```python
from build123d import *

# Parameters (mm, degrees)
SKETCH_1_R            = 1.5
EXTRUDE_1_DEPTH       = 2
SKETCH_2_R            = 0.9
SKETCH_2_W            = 62
SKETCH_2_H            = 52
CUT_EXTRUDE_1_DEPTH   = 52.264022472
EXTRUDE_START         = -2
EXTRUDE_1_2_OUTLINE_W = 34
EXTRUDE_1_2_OUTLINE_H = 16
EXTRUDE_1_2_DEPTH     = 2
SKETCH_4_R            = 3
CUT_EXTRUDE_2_DEPTH   = 52.264022472
FILLET_1_R            = 1


# Read off the part's stored shape, not the designer's step: 拉伸-薄壁1
with BuildPart() as part:
    # 草图1 → Extrude 1 (new body)
    with BuildSketch(Plane(origin=(0, 0, 0), x_dir=(1, 0, 0), z_dir=(0, 1, 0))):
        Polygon((-37, 32), (-37, 22.5), (-40, 22.5), (-40, 7.5), (-37, 7.5), (-37, -7.5), (-40, -7.5), (-40, -22.5), (-37, -22.5), (-37, -32), (37, -32), (37, -22.5), (40, -22.5), (40, -7.5), (37, -7.5), (37, 7.5), (40, 7.5), (40, 22.5), (37, 22.5), (37, 32), align=None)
        with Locations(Location((-24.5, 29, 0), (0, 0, 270))):
            Circle(SKETCH_1_R, mode=Mode.SUBTRACT)
        with Locations(Location((24.5, 29, 0), (0, 0, 90))):
            Circle(SKETCH_1_R, mode=Mode.SUBTRACT)
        with Locations(Location((24.5, -29, 0), (0, 0, 270))):
            Circle(SKETCH_1_R, mode=Mode.SUBTRACT)
        with Locations(Location((-24.5, -29, 0), (0, 0, 90))):
            Circle(SKETCH_1_R, mode=Mode.SUBTRACT)
    extrude(amount=EXTRUDE_1_DEPTH)

    # 草图2 → 切除-拉伸1 (cut, through all)
    with BuildSketch(Plane(origin=(0, 2, 0), x_dir=(1, 0, 0), z_dir=(0, 1, 0))):
        with Locations((-37, 23.4)):
            Circle(SKETCH_2_R)
        with Locations((-37, 6.6)):
            Circle(SKETCH_2_R)
        with Locations((37, 6.6)):
            Circle(SKETCH_2_R)
        with Locations((37, 23.4)):
            Circle(SKETCH_2_R)
        with Locations((37, -23.4)):
            Circle(SKETCH_2_R)
        with Locations((-37, -23.4)):
            Circle(SKETCH_2_R)
        with Locations((37, -6.6)):
            Circle(SKETCH_2_R)
        with Locations((-37, -6.6)):
            Circle(SKETCH_2_R)
        Rectangle(SKETCH_2_W, SKETCH_2_H)
    extrude(amount=-CUT_EXTRUDE_1_DEPTH, mode=Mode.SUBTRACT)

    # Extrude 1 2 outline → Extrude 1 2 (add)
    with BuildSketch(Plane(origin=(0, 2, 0), x_dir=(1, 0, 0), z_dir=(0, 1, 0)).offset(EXTRUDE_START)):
        Polygon((-31, 26), (-31, 22.666666667), (-21, 9.333333333), (-21, -9.333333333), (-31, -22.666666667), (-31, -26), (-28.5, -26), (-18, -12), (18, -12), (28.5, -26), (31, -26), (31, -22.666666667), (21, -9.333333333), (21, 9.333333333), (31, 22.666666667), (31, 26), (28.5, 26), (18, 12), (-18, 12), (-28.5, 26), align=None)
        Rectangle(EXTRUDE_1_2_OUTLINE_W, EXTRUDE_1_2_OUTLINE_H, mode=Mode.SUBTRACT)
    extrude(amount=EXTRUDE_1_2_DEPTH)

    # 草图4 → 切除-拉伸2 (cut, through all)
    with BuildSketch(Plane(origin=(0, 2, 0), x_dir=(1, 0, 0), z_dir=(0, 1, 0))):
        with Locations((-32.5, 17.8)):
            Circle(SKETCH_4_R)
        with Locations((32.5, 17.8)):
            Circle(SKETCH_4_R)
    extrude(amount=-CUT_EXTRUDE_2_DEPTH, mode=Mode.SUBTRACT)

    # 圆角1
    fillet_1_edges = [part.edges().sort_by_distance(p)[0] for p in [
        (-31, 1, -15.201923789),
        (-31, 1, -20.398076211),
        (31, 1, -20.398076211),
        (31, 1, -15.201923789),
        (37, 1, -32),
        (40, 1, -22.5),
        (40, 1, -7.5),
        (40, 1, 7.5),
        (40, 1, 22.5),
        (37, 1, 32),
        (-37, 1, 32),
        (-40, 1, 22.5),
        (-40, 1, 7.5),
        (-40, 1, -7.5),
        (-40, 1, -22.5),
        (-37, 1, -32),
    ]]
    fillet(fillet_1_edges, radius=FILLET_1_R)


solid = part.part
```
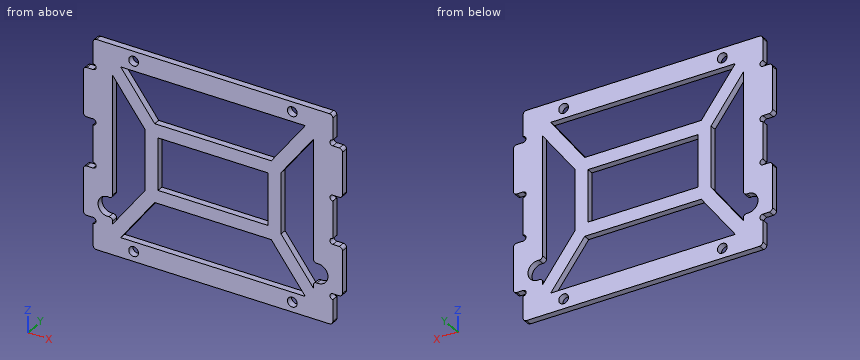
For this review, take the finished solid that the model builds, in its own axes (mm). Round coordinates to 2 decimals unless told otherwise and drop trailing zeros. Loops run counter-clockwise (first coordinate to the right, second up) from the corner with the lowest first, then second, coordinate; pieces in that order, holes last.
(1) We need section C-C (x = -27.5). Give the boundary of the cut face in (y, z).
Returned:
outline: (0, -32) - (2, -32) - (2, -26) - (0, -26) - close; (0, -24.67) - (2, -24.67) - (2, -18) - (0, -18) - close; (0, 18) - (2, 18) - (2, 24.67) - (0, 24.67) - close; (0, 26) - (2, 26) - (2, 32) - (0, 32) - close
(2) We need section B-B (z = 6.6). Give the boundary of the cut face in (x, y).
Returned:
outline: (-36.1, 0) - (-31, 0) - (-31, 2) - (-36.1, 2) - close; (-21, 0) - (-17, 0) - (-17, 2) - (-21, 2) - close; (17, 0) - (21, 0) - (21, 2) - (17, 2) - close; (31, 0) - (36.1, 0) - (36.1, 2) - (31, 2) - close
(3) Wall thickness on line 1 along Z through (x, y) = (18, 0.8); line 2 along Z through (x, y) = (6.5, 1.4); line 3 along X through (y, z) = (1, -29): over which ranges is each line inside the solid? List them lowest first.
Returned:
line 1: z = -32 to -26, -12 to 12, 26 to 32
line 2: z = -32 to -26, -12 to -8, 8 to 12, 26 to 32
line 3: x = -37 to -26, -23 to 23, 26 to 37
(4) Clearance check with flat-ended pins moving along their axes: P1, Ø1, axis at x = -38.5, y = 1.5, coming from the +Z side; P2, Ø1, axis at y = 1.5, z = 1.5, coming from the +X side; P3, Ø1, axis at x = -38, y = 0.5, coming from the -Z side. State where each tip first meets the part, or that it passes through.
Returned:
P1: stops at z = 22.5
P2: stops at x = 37
P3: stops at z = -22.5
(5) We need section D-D (y = 0.5). State how many separate pieces and enclosed holes the cut face has, plus the area to 3 significant figures.
Returned:
separate pieces: 1
enclosed holes: 9
area: 2,340 mm2
(6) We need section A-A (z = 29). Give the boundary of the cut face in (x, y), plus the area to 3 significant figures.
Returned:
outline: (-37, 0) - (-26, 0) - (-26, 2) - (-37, 2) - close; (-23, 0) - (23, 0) - (23, 2) - (-23, 2) - close; (26, 0) - (37, 0) - (37, 2) - (26, 2) - close
area: 136 mm2
